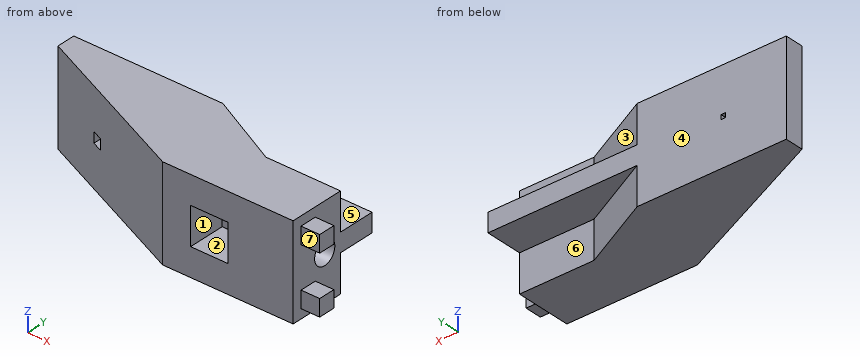
Autodesk Inventor part; units mm, degrees
ref_plane "YZ Plane" through (0, 0, 0) normal (1, 0, 0) x (0, 1, 0)
ref_plane "XZ Plane" through (0, 0, 0) normal (0, 1, 0) x (-1, 0, 0)
ref_plane "XY Plane" through (0, 0, 0) normal (0, 0, 1) x (1, 0, 0)
sketch "Sketch1" plane through (0, 0, 0) normal (1, 0, 0) x (0, 1, 0)
  line L0 (-7.5, -12.5) -> (7.5, -12.5)
  line L1 (7.5, -12.5) -> (7.5, 12.5)
  line L2 (7.5, 12.5) -> (-7.5, 12.5)
  line L3 (-7.5, 12.5) -> (-7.5, -12.5)
  line L4 (-7.5, -12.5) -> (7.5, 12.5) construction
  line L5 (7.5, -12.5) -> (-7.5, 12.5) construction
  point P0 (0, 0)
  dimension "d0" = 15
  dimension "d1" = 25
extrude "Extrusion1" add sketch "Sketch1" against normal blind 80
sketch "Sketch2" plane through (0, 0, 0) normal (1, 0, 0) x (0, 0, -1)
  line L0 (-12.5, 7.5) -> (12.5, 7.5)
  line L1 (0, 7.5) -> (2.5, 7.5)
  line L2 (2.5, 7.5) -> (2.5, 17.5)
  line L3 (2.5, 17.5) -> (0, 17.5)
  line L4 (0, 17.5) -> (0, 7.5)
  line L5 (0, 7.5) -> (-2.5, 7.5)
  line L6 (-2.5, 7.5) -> (-2.5, 17.5)
  line L7 (-2.5, 17.5) -> (0, 17.5)
  line L8 (0, 17.5) -> (0, 7.5)
  point P0 (0, 0)
  dimension "d4" = 2.5
  dimension "d5" = 10
  dimension "d6" = 2.5
  dimension "d7" = 10
extrude "Extrusion2" add sketch "Sketch2" against normal blind 80
sketch "Sketch4" plane through (0, 7.5, -2.5) normal (0, 0, -1) x (-1, 0, 0)
  line L0 (80, -15) -> (80, 0)
  line L1 (80, 0) -> (40, 0)
  line L2 (40, 0) -> (40, 10)
  line L3 (40, 10) -> (80, 10)
  line L4 (80, 10) -> (80, 0)
  point P0 (0, -7.5)
  dimension "d12" = 40
extrude "Extrusion3" add sketch "Sketch4" along normal blind 10
sketch "Sketch5" plane through (0, 7.5, -2.5) normal (0, 0, -1) x (-1, 0, 0)
  line L0 (0, 0) -> (80, 0)
  line L1 (40, 0) -> (20, 0)
  line L2 (20, 0) -> (40, 10)
  line L3 (40, 10) -> (40, 0)
  point P0 (0, -7.5)
  dimension "d15" = 20
extrude "Extrusion4" add sketch "Sketch5" along normal blind 10
sketch "Sketch6" plane through (0, 7.5, 2.5) normal (0, 0, 1) x (1, 0, 0)
  line L0 (-80, 10) -> (-40, 10)
  line L1 (-40, 10) -> (-40, 0)
  line L2 (-40, 0) -> (-80, 0)
  line L3 (-80, 0) -> (-80, 10)
  point P0 (0, -7.5)
extrude "Extrusion5" add sketch "Sketch6" along normal blind 10
sketch "Sketch7" plane through (0, 7.5, 2.5) normal (0, 0, 1) x (1, 0, 0)
  line L0 (-40, 10) -> (-40, 0)
  line L1 (-40, 0) -> (-20, 0)
  line L2 (0, 0) -> (-40, 0)
  line L3 (0, 10) -> (-40, 10)
  line L4 (-20, 0) -> (-40, 10)
  line L5 (-40, 10) -> (-40, 0)
  point P0 (0, -7.5)
  dimension "d20" = 20
extrude "Extrusion6" add sketch "Sketch7" along normal blind 10
sketch "Sketch8" plane through (0, -7.5, 12.5) normal (0, 0, 1) x (1, 0, 0)
  line L0 (0, 0) -> (-80, 0)
  line L1 (-80, 0) -> (-80, 20)
  line L2 (-80, 0) -> (-80, 25)
  line L3 (-80, 0) -> (-35, 0)
  line L4 (-35, 0) -> (-80, 20)
  point P0 (0, 7.5)
  dimension "d23" = 20
  dimension "d24" = 45
extrude "Extrusion7" cut sketch "Sketch8" against normal blind 25
sketch "Sketch21" plane through (0, 17.5, 2.5) normal (0, 1, 0) x (1, 0, 0)
  line L0 (-62.5195, 3.1) -> (-63.7195, 3.1)
  line L1 (-63.7195, 3.1) -> (-63.7195, 1.9)
  line L2 (-63.7195, 1.9) -> (-62.5195, 1.9)
  line L3 (-62.5195, 1.9) -> (-62.5195, 3.1)
  line L4 (-62.5195, 3.1) -> (-63.7195, 1.9) construction
  line L5 (-63.7195, 3.1) -> (-62.5195, 1.9) construction
  point P0 (0, 2.5)
  point P1 (-63.1195, 2.5)
  dimension "d63" = 1.2
  dimension "d64" = 1.2
extrude "Extrusion15" cut sketch "Sketch21" against normal blind 8.2
sketch "Sketch28" plane through (0, -7.5, -12.5) normal (0, -1, 0) x (1, 0, 0)
  line L0 (-17.5, 7.5) -> (-27.5, 7.5)
  line L1 (-27.5, 7.5) -> (-27.5, 17.5)
  line L2 (-27.5, 17.5) -> (-17.5, 17.5)
  line L3 (-17.5, 17.5) -> (-17.5, 7.5)
  line L4 (-17.5, 7.5) -> (-27.5, 17.5) construction
  line L5 (-27.5, 7.5) -> (-17.5, 17.5) construction
  point P0 (0, 12.5)
  point P1 (-22.5, 12.5)
  dimension "d86" = 10
  dimension "d87" = 10
extrude "Extrusion18" cut sketch "Sketch28" against normal blind 10
sketch "Sketch30" plane through (0, 0, 0) normal (1, 0, 0) x (0, 0, -1)
  line L0 (-12.5, -7.5) -> (12.5, -7.5)
  line L1 (0, -7.5) -> (0, 2.5)
  point P0 (0, 0)
  dimension "d90" = 10
hole "Hole1" at (0, 2.5, 0) direction (-1, 0, 0) diameter 6.4 depth 10 tip angle 118
sketch "Sketch31" plane through (0, 9.3, 2.5) normal (0, 1, 0) x (1, 0, 0)
  line L0 (-64.5195, 1.1) -> (-61.7195, 1.1)
  line L1 (-61.7195, 1.1) -> (-61.7195, 3.9)
  line L2 (-61.7195, 3.9) -> (-64.5195, 3.9)
  line L3 (-64.5195, 3.9) -> (-64.5195, 1.1)
  line L4 (-64.5195, 1.1) -> (-61.7195, 3.9) construction
  line L5 (-61.7195, 1.1) -> (-64.5195, 3.9) construction
  point P0 (0, 2.5)
  point P1 (-63.1195, 2.5)
  dimension "d98" = 2.8
  dimension "d99" = 2.8
extrude "Extrusion19" cut sketch "Sketch31" against normal through all
chamfer "Chamfer3" distance 0.8 angle 45 4 edges at (-62.5195, 9.3, 0) (-63.1195, 9.3, -0.6) (-63.1195, 9.3, 0.6) (-63.7195, 9.3, 0)
sketch "Sketch32" plane through (0, 0, 0) normal (1, 0, 0) x (0, 0, -1)
  line L0 (-12.5, -7.5) -> (12.5, -7.5)
  line L1 (-12.5, -7.5) -> (-10, -7.5)
  line L2 (-10, -7.5) -> (-10, -5)
  line L3 (-10, -5) -> (-12.5, -5)
  line L4 (-12.5, -5) -> (-12.5, -7.5)
  line L5 (-10, -5) -> (-5.5, -5)
  line L6 (-5.5, -5) -> (-5.5, -0.5)
  line L7 (-5.5, -0.5) -> (-10, -0.5)
  line L8 (-10, -0.5) -> (-10, -5)
  point P0 (0, 0)
  dimension "d105" = 2.5
  dimension "d106" = 2.5
  dimension "d107" = 4.5
  dimension "d108" = 4.5
extrude "Extrusion20" add sketch "Sketch32" along normal blind 5 contours L8 L7 L6 L5
sketch "Sketch33" plane through (0, 0, 0) normal (1, 0, 0) x (0, 0, -1)
  line L0 (12.5, -7.5) -> (12.5, 12.5)
  line L1 (12.5, -7.5) -> (10, -7.5)
  line L2 (10, -7.5) -> (10, -5)
  line L3 (10, -5) -> (12.5, -5)
  line L4 (12.5, -5) -> (12.5, -7.5)
  line L5 (10, -5) -> (5.5, -5)
  line L6 (5.5, -5) -> (5.5, -0.5)
  line L7 (5.5, -0.5) -> (10, -0.5)
  line L8 (10, -0.5) -> (10, -5)
  point P0 (0, 0)
  dimension "d111" = 2.5
  dimension "d112" = 2.5
  dimension "d113" = 4.5
  dimension "d114" = 4.5
extrude "Extrusion21" add sketch "Sketch33" along normal blind 5 contours L5 L6 L7 L8
properties part number "end"
Geometry: final body of the model. Coordinates: model frame, mm. Face numbers are marked on the shaded views. A direction names the side the tool comes from. Round coordinates to 2 decimals unless told otherwise and drop trailing zeros. Write each loop counter-clockwise with the first axis right and the second up, starting at its lowest first coordinate (ties: lowest second). Pieces come first, ordered by that corner, then holes.
Item 1: Section query B-B (z = -8). Return loops of the section in (x, y), plus the area to 3 significant figures.
Item 2: Section query A-A (y = 6.5). Return loops of the section in (x, z), plus the area to 3 significant figures.
Item 3: Pin query (flat end, axial travel): P1, Ø11, axis at y = -3, z = 2, coming from the -X side; P2, Ø1, axis at x = -38, z = -3, coming from the -Y side; P3, Ø2, axis at x = 1.5, y = -3.5, coming from the +Z side. Return the tip coordinate at first contact, or that it passes through.
Item 4: Section query D-D (y = 15.5). Return loops of the section in (x, z).
Item 5: Mould query, pull axis X, two halves, no side actions, for the marked faces 1, 2, 3 and 4. Classes: +X half, -X half, draft (parallel to the pull), parting line (faces both ways), or undercut.
Item 6: Section query C-C (x = -22.5). Return loops of the section in (y, z).
Item 7: Set-up query: the marked faces 5, 6 and 7. Return all of +Z, -Z, +X, -X, +Y, -Y with unobstructed straight access to the full face (end or side cutting, diameter ignored); none if empty.
Item 8: Material intervals for L1, parallel to Y at x = -2.75, z = 0; L2, parallel to Z at x = -5, y = 2.5; L3, parallel to Y at x = -16, z = 8.25, sorted ascending.
Completed:
1. outline: (-80, 12.5) - (-35, -7.5) - (0, -7.5) - (0, -5) - (5, -5) - (5, -0.5) - (0, -0.5) - (0, 7.5) - (-20, 7.5) - (-40, 17.5) - (-80, 17.5) - close
1. area: 1,270 mm2
2. outline: (-66.5, -12.5) - (0, -12.5) - (0, 12.5) - (-66.5, 12.5) - close; hole (-64.52, -1.4) - (-61.72, -1.4) - (-61.72, 1.4) - (-64.52, 1.4) - close
2. area: 1,650 mm2
3. P1: stops at x = -57.5
3. P2: stops at y = -6.39
3. P3: stops at z = 10
4. outline: (-80, -12.5) - (-36, -12.5) - (-36, -2.5) - (0, -2.5) - (0, 2.5) - (-36, 2.5) - (-36, 12.5) - (-80, 12.5) - close; hole (-63.72, -0.6) - (-62.52, -0.6) - (-62.52, 0.6) - (-63.72, 0.6) - close
5. face 1: undercut
5. face 2: undercut
5. face 3: +X half
5. face 4: draft
6. outline: (-7.5, -12.5) - (8.75, -12.5) - (8.75, -2.5) - (17.5, -2.5) - (17.5, 2.5) - (8.75, 2.5) - (8.75, 12.5) - (-7.5, 12.5) - (-7.5, 5) - (2.5, 5) - (2.5, -5) - (-7.5, -5) - close
7. face 5: +Z, +X, +Y
7. face 6: -Z, +X, +Y
7. face 7: +Z, -Z, +X, -Y
8. L1: y = -7.5 to -0.7, 5.7 to 17.5
8. L2: z = -12.5 to -3.2, 3.2 to 12.5
8. L3: y = -7.5 to 7.5
